For this review, take the finished solid that the model builds, in its own axes (mm). Face numbers are marked on the shaded views. A direction names the side the tool comes from. Coordinates: 2 decimals unless noted, no trailing zeros. Loops run counter-clockwise (first coordinate to the right, second up) from the corner with the lowest first, then second, coordinate; pieces in that order, holes last. Notation, with made-up numbers: (2, 16) -> (18, 16) arc R24 ccw to (18, 45) -> close; hole circle Ø6 at (44.25, 69.5). An arc over 180 degrees is marked (long way). One line per item, written item: value.
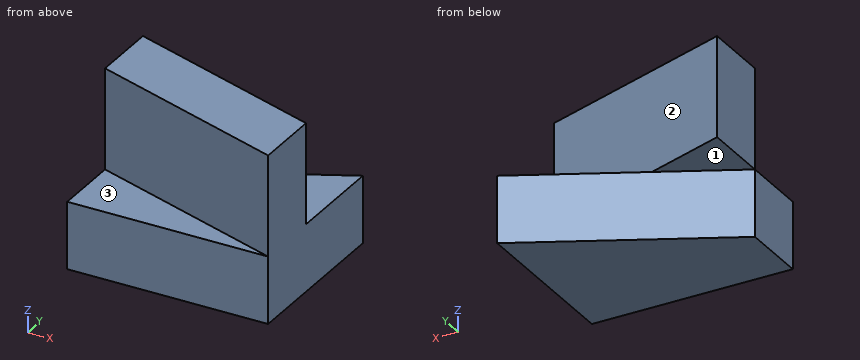
from build123d import *

# Parameters (mm, degrees)
BOSS_EXTRUDE1_DEPTH = 10
BOSS_EXTRUDE4_DEPTH = 15


with BuildPart() as part:
    # Sketch1 → Boss-Extrude1 (new body)
    with BuildSketch(Plane.XY):
        Polygon((0, 0), (-30, 0), (-30, 10), (0, 25), align=None)
    extrude(amount=BOSS_EXTRUDE1_DEPTH)

    # Sketch2 → Boss-Extrude4 (add)
    with BuildSketch(Plane.XY.offset(10)):
        Polygon((-30, 10), (0, 0), (0, 10), (-30, 20), align=None)
    extrude(amount=BOSS_EXTRUDE4_DEPTH)


solid = part.part
1. To check wall thickness, follow probe 1 along Z at (x, y) = (-29, 4.25); probe 2 along Y at (x, z) = (-23.5, 7); probe 3 along Y at (x, z) = (-19, 15). State the ranges of each line that lie inside material, in increasing order. Write a range as from..to.
Return value:
probe 1: z = 0..10
probe 2: y = 0..13.25
probe 3: y = 6.33..16.33
2. Insertion check: pin 1 Ø2 at (x, z) = (-25.5, 17) entering from -Y; pin 2 Ø2 at (x, z) = (-26.5, 15.5) entering from -Y; pin 3 Ø1.5 at (x, z) = (-8, 19.5) entering from -Y; pin 4 Ø12 at (x, y) = (-7, 18.5) entering from +Z. Each pin has a flat end and moves straight along its axis. Give the tip position at first contact, or say it passes through.
Return value:
pin 1: stops at y = 8.17
pin 2: stops at y = 8.5
pin 3: stops at y = 2.42
pin 4: stops at z = 25
3. Take a section at C-C, the plane y = 11.75. Give the boundary of the cut face in (x, z), and give its area (3 significant figures).
Return value:
outline: (-30, 10) -> (-26.5, 10) -> (-26.5, 0) -> (0, 0) -> (0, 10) -> (-5.25, 10) -> (-5.25, 25) -> (-30, 25) -> close
area: 636 mm2
4. For the marked faces 1, 2 and 3, list the 3-axis set-ups (+Z, -Z, +X, -X, +Y, -Y) from which the entire face can be reached by the end or side of a thin tool; tool diameter is ignored.
Return value:
face 1: -Z, -X, +Y
face 2: +Z, +X, +Y
face 3: +Z, -X, -Y
5. Take a section at D-D, the plane z = 23. Give the boundary of the cut face in (x, y), and give its area (3 significant figures).
Return value:
outline: (-30, 10) -> (0, 0) -> (0, 10) -> (-30, 20) -> close
area: 300 mm2
6. Take a section at A-A, the plane y = 16.5. Give the boundary of the cut face in (x, z), and give its area (4 significant figures).
Return value:
outline: (-30, 10) -> (-19.5, 10) -> (-19.5, 25) -> (-30, 25) -> close; (-17, 0) -> (0, 0) -> (0, 10) -> (-17, 10) -> close
area: 327.5 mm2
7. Take a section at B-B, the plane x = -25.5. Give the boundary of the cut face in (y, z).
Return value:
outline: (0, 0) -> (12.25, 0) -> (12.25, 10) -> (18.5, 10) -> (18.5, 25) -> (8.5, 25) -> (8.5, 10) -> (0, 10) -> close
